CAD build for the part. Positions are in the model's coordinates, mm. A direction names the side the tool comes from. Give positions to 0.01 mm unless a question says otherwise; leave off trailing zeros. Loops run counter-clockwise (first coordinate to the right, second up) from the corner with the lowest first, then second, coordinate; pieces in that order, holes last. Notation, with made-up numbers: M 85.25,70.5 L 95.25,70.5 A18 ccw 95.25,104.5 Z; hole C 77.25,87 d8. An arc over 180 degrees is marked long. One line per question, with ' | ' between items.
```python
from build123d import *

# Parameters (mm, degrees)
F0_W           = 139.7
F0_H           = 88.9
F0_W_2         = 63.5
F0_H_2         = 34.925
F1_DEPTH       = 12.7
F2_W           = 9.525
F2_H           = 9.525
F2_W_2         = 69.85
F2_H_2         = 41.275
F3_DEPTH       = 9.525
F4_W           = 33.02
F4_H           = 13.97
F5_DEPTH       = 6.35
F7_D           = 6.35
F7_CBORE_D     = 12.7
F7_CBORE_DEPTH = 6.35


with BuildPart() as f1:
    # F0 (on Top) → F1 (new body)
    with BuildSketch(Plane.XY):
        with Locations((-69.85, -44.45)):
            Rectangle(F0_W, F0_H)
        with Locations((-50.8, -58.7375)):
            Rectangle(F0_W_2, F0_H_2, mode=Mode.SUBTRACT)
    extrude(amount=F1_DEPTH)

    # F2 (on face) → F3 (cut)
    with BuildSketch(Plane(origin=(0, 0, 0), x_dir=(1, 0, 0), z_dir=(0, 0, -1))):
        with Locations((-131.7625, 7.9375)):
            Rectangle(F2_W, F2_H)
        with Locations((-131.7625, 80.9625)):
            Rectangle(F2_W, F2_H)
        with Locations((-7.9375, 7.9375)):
            Rectangle(F2_W, F2_H)
        with Locations((-7.9375, 80.9625)):
            Rectangle(F2_W, F2_H)
        with Locations((-50.8, 58.7375)):
            Rectangle(F2_W_2, F2_H_2)
    extrude(amount=-F3_DEPTH, mode=Mode.SUBTRACT)

    # F4 (on face) → F5 (cut)
    with BuildSketch(Plane.XY.offset(12.7)):
        with Locations((-32.385, -22.86)):
            Rectangle(F4_W, F4_H)
    extrude(amount=-F5_DEPTH, mode=Mode.SUBTRACT)

    # F7 (through all)
    with Locations(Plane(origin=(0, 0, 0), x_dir=(1, 0, 0), z_dir=(0, 0, -1))):
        with Locations((-111.960039, 60.325)):
            CounterBoreHole(F7_D / 2, F7_CBORE_D / 2, F7_CBORE_DEPTH)


solid = f1.part
```
Item 1: Saw through at A-A on x = -66. Give the cut face in (y, z) (3 decimals).
Conclusion:
outline: M -88.9,0 L -79.375,0 L -79.375,9.525 L -76.2,9.525 L -76.2,12.7 L -88.9,12.7 Z; M -41.275,9.525 L -38.1,9.525 L -38.1,0 L 0,0 L 0,12.7 L -41.275,12.7 Z
Item 2: Saw through at B-B on y = -19. Give the cut face in (x, z) (3 decimals).
Conclusion:
outline: M -139.7,0 L 0,0 L 0,12.7 L -15.875,12.7 L -15.875,6.35 L -48.895,6.35 L -48.895,12.7 L -139.7,12.7 Z
Item 3: 3-axis set-ups, long thin cutter, end or side, ignore diameter. For faces 1 (the flat face through (-71, -88.9, 6)), 2 (the flat face through (-51, -41.275, 11)), 3 (the flat face through (-51, -79.375, 5)), 4 (the flat face through (-33, -23, 6.35)): which of +Z, -Z, +X, -X, +Y, -Y reach the whole face in a straight line?
Conclusion:
face 1: +Z, -Z, +X, -X, -Y | face 2: +Z, -Z | face 3: -Z | face 4: +Z
Item 4: Mould opens along Y. For faces 5 (the flat face through (-71, 0, 6)), 6 (the flat face through (-71, -34, 0)), 7 (the flat face through (-127, -81, 5)) say: pulls with the +Y half, pulls with the -Y half, needs draft (parallel to the pull), parting line crosses it, or undercut.
Conclusion:
face 5: pulls with the +Y half | face 6: needs draft | face 7: undercut
Item 5: Drill centre lines: line 1 along X through (y, z) = (-5, 2) (3 decimals); line 2 along Y through (x, z) = (-36, 8) (3 decimals); line 3 along X through (y, z) = (-70.5, 8.25) (3 decimals). Where is each one in solid material? Low to high. Write a range as [from, to].
Conclusion:
line 1: [-139.7, -136.525], [-127, -12.7], [-3.175, 0] | line 2: [-88.9, -79.375], [-38.1, -29.845], [-15.875, 0] | line 3: [-139.7, -85.725], [-15.875, 0]
Item 6: Saw through at C-C on x = -130. Give the cut face in (y, z) (3 decimals).
Conclusion:
outline: M -88.9,0 L -85.725,0 L -85.725,9.525 L -76.2,9.525 L -76.2,0 L -12.7,0 L -12.7,9.525 L -3.175,9.525 L -3.175,0 L 0,0 L 0,12.7 L -88.9,12.7 Z
Item 7: Drop flat-ended pins along their axis: P1, Ø5, axis at x = -6, z = 4.5, coming from the +Y side; P2, Ø3, axis at x = -7.5, y = -80, coming from the -Z side (3 decimals). Give the stop position or say it passes through.
Conclusion:
P1: y = 0 | P2: z = 9.525
Item 8: Saw through at D-D on z = 4. Give the cut face in (x, y) (3 decimals), and give its area (3 significant figures).
Conclusion:
outline: M -139.7,-88.9 L 0,-88.9 L 0,0 L -139.7,0 Z; hole M -136.525,-85.725 L -127,-85.725 L -127,-76.2 L -136.525,-76.2 Z; hole M -136.525,-12.7 L -127,-12.7 L -127,-3.175 L -136.525,-3.175 Z; hole C -111.96,-60.325 d12.7; hole M -85.725,-79.375 L -15.875,-79.375 L -15.875,-38.1 L -85.725,-38.1 Z; hole M -12.7,-85.725 L -3.175,-85.725 L -3.175,-76.2 L -12.7,-76.2 Z; hole M -12.7,-12.7 L -3.175,-12.7 L -3.175,-3.175 L -12.7,-3.175 Z | area: 9,050 mm²
